For this review, take the finished solid that the model builds, in its own axes (mm). Face numbers are marked on the shaded views. A direction names the side the tool comes from. Give positions to 0.01 mm unless a question says otherwise; leave off trailing zeros. Write each loop counter-clockwise with the first axis right and the second up, starting at its lowest first coordinate (ties: lowest second). Pieces come first, ordered by that corner, then holes. Notation, with made-up numbers: M 39.5,-2.75 L 61.5,-2.75 A18 ccw 61.5,14.25 Z; hole C -29,-34.75 d5. An arc over 180 degrees is marked long. One line per item, written item: value. Start each with the question number.
Item 1: Consider section C-C, the plane x = -74.5. Write out the cut boundary in (y, z).
Item 2: Consider section B-B, the plane z = 27. Write out the cut boundary in (x, y), and give its area (3 significant figures).
Item 3: To check wall thickness, follow probe 1 along Z at (x, y) = (-48, -27.5); probe 2 along Y at (x, z) = (-81, 34.5); probe 3 along X at (y, z) = (-6, 31). State the ranges of each line that lie inside material, in increasing order.
Item 4: Mouldability with a two-part tool opening along Z and no side actions: class the marked faces 4, 5, 6 and 7 as released by +Z, released by -Z, zero draft, split by the parting line, or undercut.
Item 5: Tool access review of the marked faces 1, 2 and 3: name each direction out of +Z, -Z, +X, -X, +Y, -Y from which nothing blocks a thin tool from reaching the whole face with its end or side.
Item 6: Consider section D-D, the plane y = -21. Write out the cut boundary in (x, z), and give its area (3 significant figures).
Item 7: Consider section A-A, the plane y = -6. Write out the cut boundary in (x, z).
Item 8: Clearance check with flat-ended pins moving along their axes: pin 1 Ø3 at (y, z) = (-7, 35) entering from -X; pin 2 Ø8 at (x, y) = (-64, -11) entering from +Z; pin 3 Ø4 at (x, y) = (-67, -4) entering from +Z. State where each tip first meets the part, or that it passes through.
```python
from build123d import *

# Parameters (mm, degrees)
F0_W      = 63.5
F0_H      = 6.35
F1_DEPTH  = 38.1
F3_DEPTH  = 25.4
F5_DEPTH  = 25.4
F6_W      = 25.4
F6_H      = 25.4
F7_DEPTH  = 12.7
F9_DEPTH  = 12.7
F11_DEPTH = 12.7
F12_R     = 6.35
F13_DEPTH = 25.4


with BuildPart() as f1:
    # F0 (on Front) → F1 (new body)
    with BuildSketch(Plane.XZ):
        with Locations((-55.4636918637, 3.175)):
            Rectangle(F0_W, F0_H)
    extrude(amount=F1_DEPTH)

    # F2 (on face) → F3 (cut)
    with BuildSketch(Plane.XY.offset(6.35)):
        with BuildLine():
            ThreePointArc((-23.7136918637, -26.2837559164), (-27.2983828623, -34.5153090014), (-35.5299359473, -38.1))
            Line((-35.5299359473, -38.1), (-23.7136918637, -38.1))
            Line((-23.7136918637, -38.1), (-23.7136918637, -26.2837559164))
        make_face()
    extrude(amount=-F3_DEPTH, mode=Mode.SUBTRACT)

    # F4 (on face) → F5 (cut)
    with BuildSketch(Plane.XY.offset(6.35)):
        with BuildLine():
            ThreePointArc((-73.6299359473, -38.1), (-82.2750994664, -33.7322502916), (-87.2136918637, -25.4))
            Line((-87.2136918637, -25.4), (-87.2136918637, -38.1))
            Line((-87.2136918637, -38.1), (-73.6299359473, -38.1))
        make_face()
    extrude(amount=-F5_DEPTH, mode=Mode.SUBTRACT)

    # F6 (on face) → F7 (join)
    with BuildSketch(Plane(origin=(0, 0, 0), x_dir=(-1, 0, 0), z_dir=(0, 1, 0))):
        with Locations((74.5136918637, 19.05)):
            Rectangle(F6_W, F6_H)
    extrude(amount=-F7_DEPTH)

    # F8 (on face) → F9 (join)
    with BuildSketch(Plane(origin=(0, 0, 0), x_dir=(-1, 0, 0), z_dir=(0, 1, 0))):
        with BuildLine():
            ThreePointArc((61.8136918637, 19.05), (57.5939587617, 10.569733102), (49.1136918637, 6.35))
            Line((49.1136918637, 6.35), (61.8136918637, 6.35))
            Line((61.8136918637, 6.35), (61.8136918637, 19.05))
        make_face()
    extrude(amount=-F9_DEPTH)

    # F10 (on face) → F11 (join)
    with BuildSketch(Plane(origin=(0, 0, 0), x_dir=(-1, 0, 0), z_dir=(0, 1, 0))):
        with BuildLine():
            Line((61.8136918637, 31.75), (87.2136918637, 31.75))
            ThreePointArc((87.2136918637, 31.75), (74.5136918637, 44.45), (61.8136918637, 31.75))
        make_face()
    extrude(amount=-F11_DEPTH)

    # F12 (on face) → F13 (cut)
    with BuildSketch(Plane.XZ.offset(12.7)):
        with Locations((-74.5136918637, 31.75)):
            Circle(F12_R)
    extrude(amount=-F13_DEPTH, mode=Mode.SUBTRACT)


solid = f1.part
```
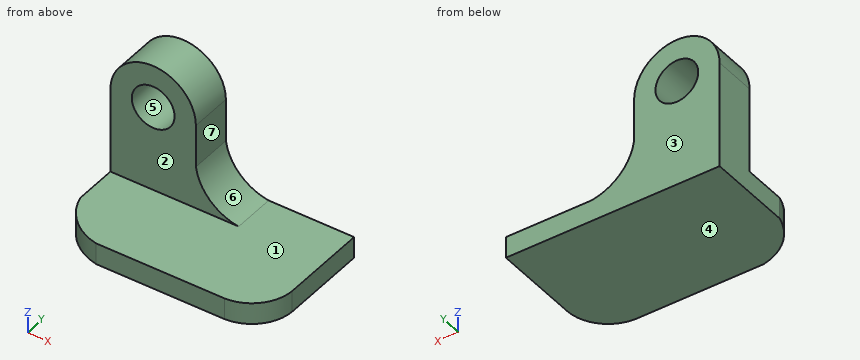
Model answer:
1. outline: M -37.91,0 L 0,0 L 0,25.4 L -12.7,25.4 L -12.7,6.35 L -37.91,6.35 Z; M -12.7,38.1 L 0,38.1 L 0,44.45 L -12.7,44.45 Z
2. outline: M -87.21,-12.7 L -78.73,-12.7 L -78.73,0 L -87.21,0 Z; M -70.3,-12.7 L -61.81,-12.7 L -61.81,0 L -70.3,0 Z
2. area: 216 mm2
3. probe 1: z = 0 to 6.35
3. probe 2: y = -12.7 to 0
3. probe 3: x = -87.21 to -80.82, -68.21 to -61.81
4. face 4: released by -Z
4. face 5: undercut
4. face 6: released by +Z
4. face 7: zero draft
5. face 1: +Z, +X, -Y
5. face 2: +Z, +X, -X, -Y
5. face 3: +Z, -Z, +X, -X, +Y
6. outline: M -87.21,0 L -23.71,0 L -23.71,6.35 L -87.21,6.35 Z
6. area: 403 mm2
7. outline: M -87.21,0 L -23.71,0 L -23.71,6.35 L -49.11,6.35 A14.89 cw -61.81,19.05 L -61.81,31.75 A12.7 ccw -87.21,31.75 Z; hole C -74.51,31.75 d12.7
8. pin 1: stops at x = -87.09
8. pin 2: stops at z = 42.65
8. pin 3: stops at z = 43.19
